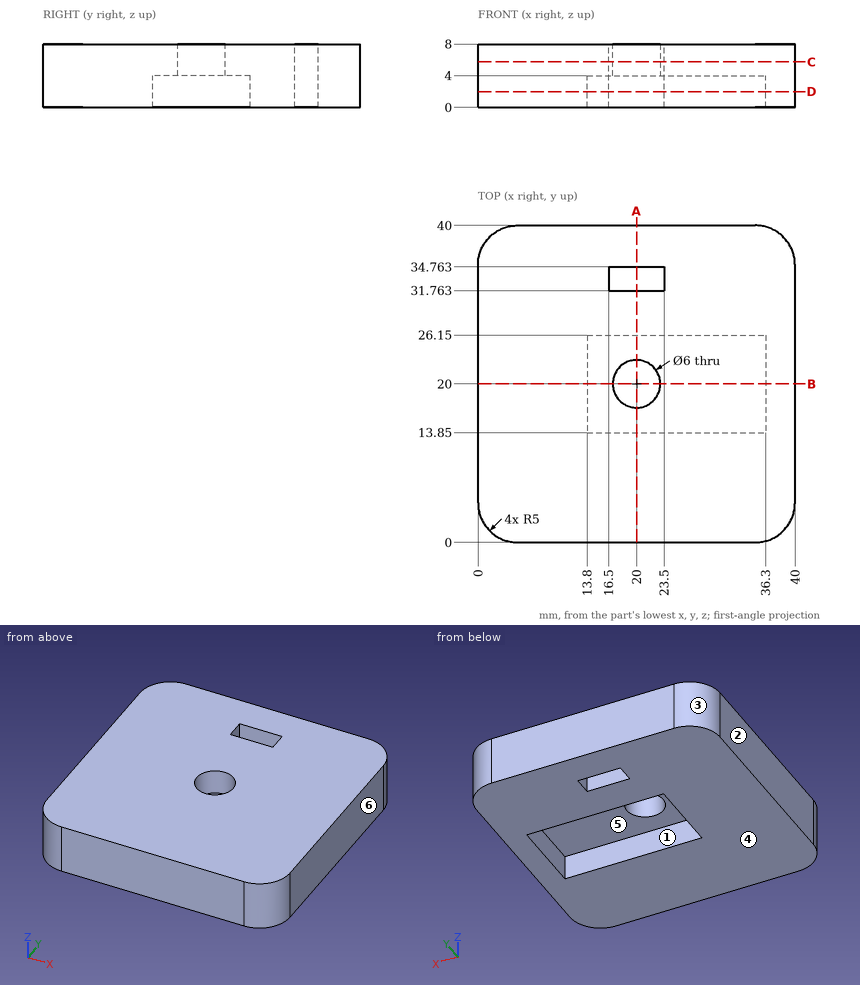
Could you check a few things on this drawing? It's one solid part, dimensions in mm from its lowest x, y, z. A direction names the side the tool comes from. Coordinates: 2 decimals unless noted, no trailing zeros. Loops run counter-clockwise (first coordinate to the right, second up) from the corner with the lowest first, then second, coordinate; pieces in that order, holes last. Notation, with made-up numbers: (-30.75, -22.5) - (12.25, -22.5) arc R14 ccw to (12.25, -6.5) - close; hole circle Ø8 at (43, 76). An arc over 180 degrees is marked (long way). Return JSON: item names as keys, results as strings. Group by question number.
Item 1: On a 3-axis mill with a long thin cutter (end or side, diameter ignored), from which of +Z, -Z, +X, -X, +Y, -Y can I reach the whole of each face in a straight line? I mean the marked faces 1 and 2. Say none if no direction works.
Item 2: If we section it at C-C on z = 5.75: Write out the boundary of the cut face in (x, y).
Item 3: Will this pin go through, and if not, where does the flat tip stop? P1, Ø5.5, axis at x = 20, y = 20, coming from the -Z side.
Item 4: If we section it at A-A on x = 20: Write out the boundary of the cut face in (y, z), and give its area (3 significant figures).
Item 5: We'd pull the mould along X, two halves only. Please class the marked faces 3, 4, 5 and 6: +X half, -X half, draft (parallel to the pull), parting line (faces both ways), or undercut.
Item 6: I need wall thicknesses on line 1 (Y direction, x = 20, z = 5.5); line 2 (Y direction, x = 33.5, z = 3.25); line 3 (Z direction, x = 32, y = 24.5). Which ranges of each line are inside material? Lowest first, please. Write a range as from..to.
Item 7: If we section it at B-B on y = 20: Write out the boundary of the cut face in (x, z), and give its area (3 significant figures).
Item 8: If we section it at D-D on z = 2: Write out the boundary of the cut face in (x, y).
Calculated:
{
 "1": {"face 1": "-Z", "face 2": "+Z, -Z, -X, +Y, -Y"},
 "2": {"outline": "(0, 5) arc R5 ccw to (5, 0) - (35, 0) arc R5 ccw to (40, 5) - (40, 35) arc R5 ccw to (35, 40) - (5, 40) arc R5 ccw to (0, 35) - close; hole (16.5, 31.76) - (23.5, 31.76) - (23.5, 34.76) - (16.5, 34.76) - close; hole circle Ø6 at (20, 20)"},
 "3": {"P1": "passes through"},
 "4": {"outline": "(0, 0) - (13.85, 0) - (13.85, 4) - (17, 4) - (17, 8) - (0, 8) - close; (23, 4) - (26.15, 4) - (26.15, 0) - (31.76, 0) - (31.76, 8) - (23, 8) - close; (34.76, 0) - (40, 0) - (40, 8) - (34.76, 8) - close", "area": "223 mm^2"},
 "5": {"face 3": "-X half", "face 4": "draft", "face 5": "undercut", "face 6": "+X half"},
 "6": {"line 1": "y = 0..17, 23..31.76, 34.76..40", "line 2": "y = 0..13.85, 26.15..40", "line 3": "z = 4..8"},
 "7": {"outline": "(0, 0) - (13.8, 0) - (13.8, 4) - (17, 4) - (17, 8) - (0, 8) - close; (23, 4) - (36.3, 4) - (36.3, 0) - (40, 0) - (40, 8) - (23, 8) - close", "area": "206 mm^2"},
 "8": {"outline": "(0, 5) arc R5 ccw to (5, 0) - (35, 0) arc R5 ccw to (40, 5) - (40, 35) arc R5 ccw to (35, 40) - (5, 40) arc R5 ccw to (0, 35) - close; hole (13.8, 13.85) - (36.3, 13.85) - (36.3, 26.15) - (13.8, 26.15) - close; hole (16.5, 31.76) - (23.5, 31.76) - (23.5, 34.76) - (16.5, 34.76) - close"}
}
